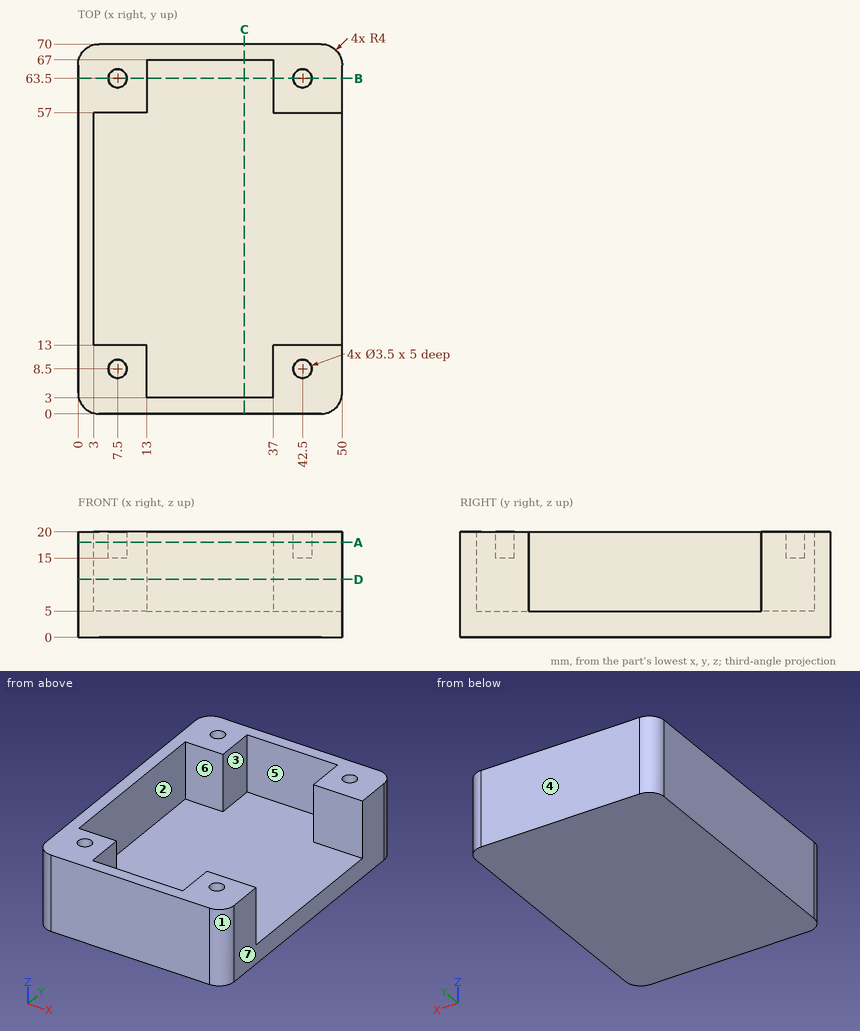
Study the drawing (mm; zero at the part's minimum x, y, z) and answer. A direction names the side the tool comes from. Give positions to 0.01 mm unless a question says otherwise; leave off trailing zeros. Loops run counter-clockwise (first coordinate to the right, second up) from the corner with the lowest first, then second, coordinate; pieces in that order, holes last. Notation, with made-up numbers: M 40,61.5 L 53,61.5 A19 cw 53,69.5 Z; hole C 83,54 d10. An arc over 180 degrees is marked long. One line per item, written item: value.
1. Find the intervals of material crossed by probe 1 along X at (y, z) = (8.5, 18.35); probe 2 along Y at (x, z) = (42.5, 18.3); probe 3 along Y at (x, z) = (38, 14.5), in increasing order.
Found:
probe 1: 0 to 5.75, 9.25 to 13, 37 to 40.75, 44.25 to 50
probe 2: 0 to 6.75, 10.25 to 13, 57 to 61.75, 65.25 to 70
probe 3: 0 to 13, 57 to 70
2. For a pull along Y with two mould halves and no side action, classify the marked faces 1, 2, 3 and 4 as pulls with the +Y half, pulls with the -Y half, needs draft (parallel to the pull), parting line crosses it, or undercut.
Found:
face 1: pulls with the -Y half
face 2: undercut
face 3: undercut
face 4: pulls with the +Y half
3. Section A-A on z = 18 is taken. Determine the outline of the cut face in (x, y), plus the area to 3 significant figures.
Found:
outline: M 0,4 A4 ccw 4,0 L 46,0 A4 ccw 50,4 L 50,13 L 37,13 L 37,3 L 13,3 L 13,13 L 3,13 L 3,57 L 13,57 L 13,67 L 37,67 L 37,57 L 50,57 L 50,66 A4 ccw 46,70 L 4,70 A4 ccw 0,66 Z; hole C 7.5,8.5 d3.5; hole C 7.5,63.5 d3.5; hole C 42.5,8.5 d3.5; hole C 42.5,63.5 d3.5
area: 900 mm^2
4. For the marked faces 5, 6 and 7, determine the directions among +Z, -Z, +X, -X, +Y, -Y from which every point of the face is accessible in a straight line to the end or side of a thin tool.
Found:
face 5: +Z
face 6: +Z, +X
face 7: +Z, -Z, +X, +Y, -Y
5. Section B-B on y = 63.5 is taken. Determine the outline of the cut face in (x, z).
Found:
outline: M 0,0 L 50,0 L 50,20 L 44.25,20 L 44.25,15 L 40.75,15 L 40.75,20 L 37,20 L 37,5 L 13,5 L 13,20 L 9.25,20 L 9.25,15 L 5.75,15 L 5.75,20 L 0,20 Z
6. Section C-C on x = 31.5 is taken. Determine the outline of the cut face in (y, z).
Found:
outline: M 0,0 L 70,0 L 70,20 L 67,20 L 67,5 L 3,5 L 3,20 L 0,20 Z
7. Each of these flat-tipped pins is pushed along its axis until it touches: P1, Ø10.5, axis at x = 43, z = 9, coming from the -Y side; P2, Ø3, axis at x = 31, y = 59.5, coming from the +Z side; P3, Ø4, axis at y = 53.5, z = 14.5, coming from the +X side; P4, Ø3, axis at x = 42.5, y = 63.5, coming from the +Z side. Where does it stop, or does it pass through?
Found:
P1: y = 0
P2: z = 5
P3: x = 3
P4: z = 15
8. Section D-D on z = 11 is taken. Determine the outline of the cut face in (x, y).
Found:
outline: M 0,4 A4 ccw 4,0 L 46,0 A4 ccw 50,4 L 50,13 L 37,13 L 37,3 L 13,3 L 13,13 L 3,13 L 3,57 L 13,57 L 13,67 L 37,67 L 37,57 L 50,57 L 50,66 A4 ccw 46,70 L 4,70 A4 ccw 0,66 Z
